Design review of the part built by this model. Coordinates are the model's own, in mm. Face numbers are marked on the shaded views. A direction names the side the tool comes from. Coordinates: 2 decimals unless noted, no trailing zeros. Write each loop counter-clockwise with the first axis right and the second up, starting at its lowest first coordinate (ties: lowest second). Pieces come first, ordered by that corner, then holes. Notation, with made-up numbers: (37, 2) -> (78, 2) arc R13 ccw to (78, 15) -> close; hole circle Ø6 at (-33, 35.25). An arc over 180 degrees is marked (long way). Answer in a Markdown table with one row per item. Add a question column.
Item 1: Take a section at C-C, the plane x = 27. Write out the cut boundary in (y, z).
Item 2: Draft analysis for pull direction X (two halves, no side actions). For the marked faces 4, 5 and 6, state which applies: released by +X, released by -X, zero draft, split by the parting line, or undercut.
Item 3: Clearance check with flat-ended pins moving along their axes: P1, Ø2, axis at x = 30, y = -5, coming from the -Z side; P2, Ø10, axis at y = 18, z = 18.5, coming from the -X side; P3, Ø10, axis at x = -4, y = -1.5, coming from the +Z side. State where each tip first meets the part, or that it passes through.
Item 4: Take a section at D-D, the plane y = 25.5. Write out the cut boundary in (x, z).
Item 5: To check wall thickness, follow line 1 (Y direction, x = 0, z = 6); line 2 (Z direction, x = 6, y = 2.5); line 3 (Y direction, x = -18, z = 2). State the ranges of each line that lie inside material, in increasing order.
Item 6: Take a section at A-A, the plane x = 0. Write out the cut boundary in (y, z).
Item 7: For the marked faces 1, 2 and 3, list the 3-axis set-ups (+Z, -Z, +X, -X, +Y, -Y) from which the entire face can be reached by the end or side of a thin tool; tool diameter is ignored.
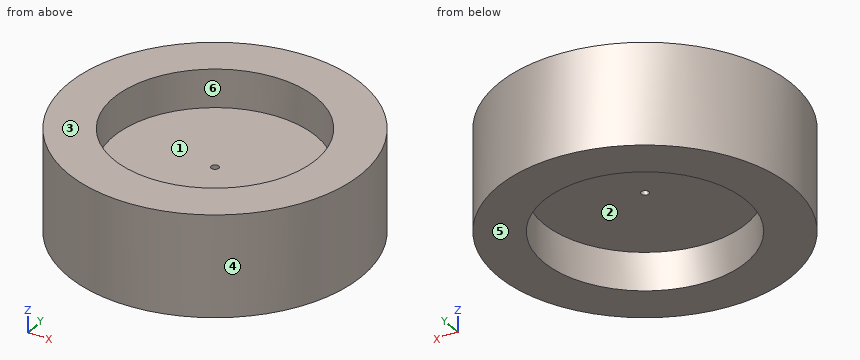
Autodesk Inventor part; units mm, degrees
ref_plane "Work Plane1" through (0, 0, 20) normal (0, 0, 1) x (1, 0, 0)
ref_plane "YZ Plane" through (0, 0, 0) normal (1, 0, 0) x (0, 1, 0)
ref_plane "XZ Plane" through (0, 0, 0) normal (0, 1, 0) x (-1, 0, 0)
sketch "Sketch1" plane through (0, 0, 0) normal (0, 0, 1) x (1, 0, 0)
  circle A0 centre (0, 0) radius 40
  circle A1 centre (0, 0) radius 58
  dimension "d0" = 80
  dimension "d2" = 116
extrude "Extrusion1" add sketch "Sketch1" along normal blind 40
ref_plane "Work Plane1" through (0, 0, 20) normal (0, 0, 1) x (1, 0, 0)
sketch "Sketch2" plane through (0, 0, 20) normal (0, 0, 1) x (1, 0, 0)
  circle A0 centre (0, 0) radius 40
extrude "Extrusion2" add sketch "Sketch2" along normal mid plane 10
sketch "Sketch3" plane through (0, 0, 15) normal (0, 0, -1) x (-1, 0, 0)
  circle A0 centre (0, 0) radius 40
  circle A1 centre (0, 0) radius 1.5
  dimension "d8" = 3
extrude "Extrusion3" cut sketch "Sketch3" against normal through all contours A1
properties part number "roda sim"
Answers:
| question | item | result |
|---|---|---|
| 1 | outline | (-51.33, 0) -> (-29.51, 0) -> (-29.51, 15) -> (29.51, 15) -> (29.51, 0) -> (51.33, 0) -> (51.33, 40) -> (29.51, 40) -> (29.51, 25) -> (-29.51, 25) -> (-29.51, 40) -> (-51.33, 40) -> close |
| 2 | face 4 | split by the parting line |
| 2 | face 5 | zero draft |
| 2 | face 6 | undercut |
| 3 | P1 | stops at z = 15 |
| 3 | P2 | stops at x = -56.52 |
| 3 | P3 | stops at z = 25 |
| 4 | outline | (-52.09, 0) -> (-30.82, 0) -> (-30.82, 15) -> (30.82, 15) -> (30.82, 0) -> (52.09, 0) -> (52.09, 40) -> (30.82, 40) -> (30.82, 25) -> (-30.82, 25) -> (-30.82, 40) -> (-52.09, 40) -> close |
| 5 | line 1 | y = -58 to -40, 40 to 58 |
| 5 | line 2 | z = 15 to 25 |
| 5 | line 3 | y = -55.14 to -35.72, 35.72 to 55.14 |
| 6 | outline | (-58, 0) -> (-40, 0) -> (-40, 15) -> (-1.5, 15) -> (-1.5, 25) -> (-40, 25) -> (-40, 40) -> (-58, 40) -> close; (1.5, 15) -> (40, 15) -> (40, 0) -> (58, 0) -> (58, 40) -> (40, 40) -> (40, 25) -> (1.5, 25) -> close |
| 7 | face 1 | +Z |
| 7 | face 2 | -Z |
| 7 | face 3 | +Z, +X, -X, +Y, -Y |
